Print and shaded views of the part. All mm, measured from the part's lowest x, y and z. Coordinates: 2 decimals unless noted, no trailing zeros. Order: outer loops, then holes, each group sorted by start corner. A loop starts at its lowest first (then second) coordinate and runs counter-clockwise, first axis right, second up. Notation, with made-up numbers: (-6, 85.25) -> (8, 85.25) arc R20 ccw to (8, 92.25) -> close; hole circle Ø2 at (87, -2.75). An arc over 180 degrees is marked (long way). Write item = value, one per line. Start each with the question number.
Q1. Cut at A-A, the plane z = 2.65. List the corners of the cut face in (x, y), plus the area to 3 significant figures.
Q2. Cut at C-C, the plane y = 20. List the corners of the cut face in (x, z).
Q3. Flat gauge pins, fed straight in: pin 1 (3 mm diameter, centred on x = 6.5, y = 7, fed in from +Z); pin 2 (1 mm diameter, centred on y = 12.5, z = 1.5, fed in from +X); pin 3 (3 mm diameter, centred on x = 38.5, y = 37, fed in from +Z); pin 4 (1 mm diameter, centred on x = 7, z = 3, fed in from +Y). Where does each tip first touch, or does it go through?
Q4. Cut at B-B, the plane x = 28. List the corners of the cut face in (y, z).
Q5. Wall check: line 1 (Z direction, x = 4.5, y = 4.5); line 2 (Y direction, x = 22, z = 2.8); line 3 (Y direction, x = 37, z = 2.15) (1 decimal). Give the ranges that are in metal, low to high. Write a range as from..to.
Q6. Cut at D-D, the plane y = 37.5. List the corners of the cut face in (x, z), plus the area to 3 significant figures.
Q7. Mould opens along Y. For the marked faces 1, 2 and 3 say: +Y half, -Y half, draft (parallel to the pull), parting line (faces both ways), or undercut.
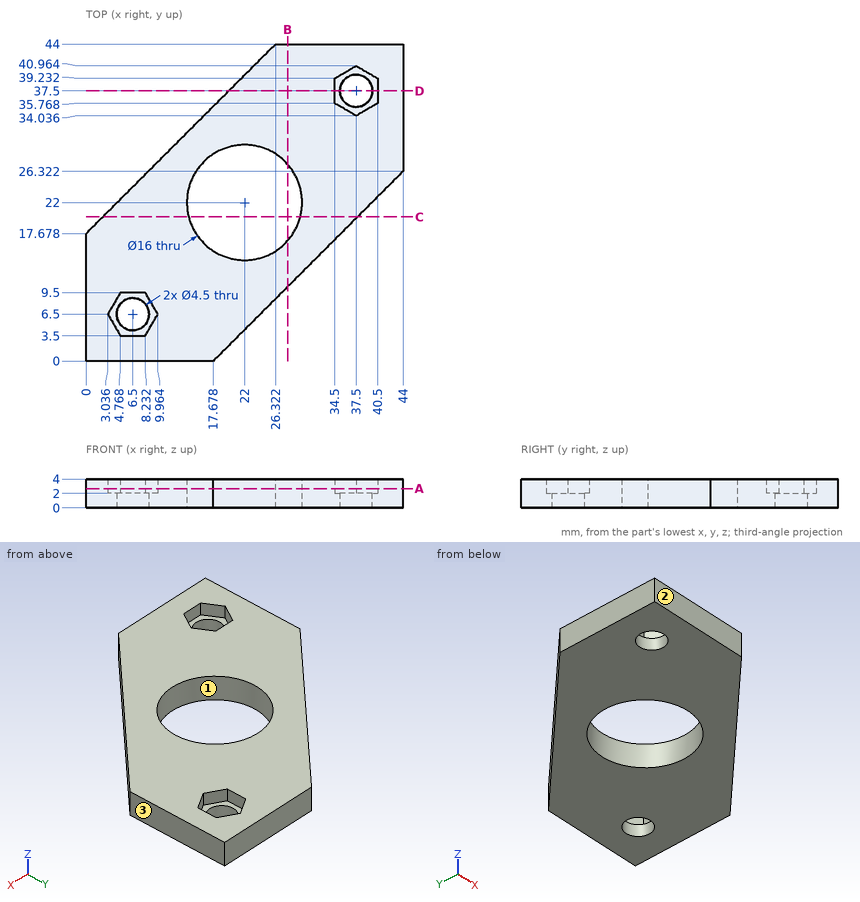
Here are the results:
q1.outline = (0, 0) -> (17.68, 0) -> (44, 26.32) -> (44, 44) -> (26.32, 44) -> (0, 17.68) -> close; hole (3.04, 6.5) -> (4.77, 3.5) -> (8.23, 3.5) -> (9.96, 6.5) -> (8.23, 9.5) -> (4.77, 9.5) -> close; hole circle Ø16 at (22, 22); hole (34.5, 35.77) -> (37.5, 34.04) -> (40.5, 35.77) -> (40.5, 39.23) -> (37.5, 40.96) -> (34.5, 39.23) -> close
q1.area = 980 mm²
q2.outline = (2.32, 0) -> (14.25, 0) -> (14.25, 4) -> (2.32, 4) -> close; (29.75, 0) -> (37.68, 0) -> (37.68, 4) -> (29.75, 4) -> close
q3.pin_1 = through
q3.pin_2 = 30.68
q3.pin_3 = 2
q3.pin_4 = 25.18
q4.outline = (10.32, 0) -> (16.71, 0) -> (16.71, 4) -> (10.32, 4) -> close; (27.29, 0) -> (44, 0) -> (44, 4) -> (27.29, 4) -> close
q5.line_1 = 0..2
q5.line_2 = 4.32..14, 30..39.68
q5.line_3 = 19.3..34.3, 40.7..44
q6.outline = (19.82, 0) -> (35.25, 0) -> (35.25, 2) -> (34.5, 2) -> (34.5, 4) -> (19.82, 4) -> close; (39.75, 0) -> (44, 0) -> (44, 4) -> (40.5, 4) -> (40.5, 2) -> (39.75, 2) -> close
q6.area = 75.7 mm²
q7.face_1 = undercut
q7.face_2 = -Y half
q7.face_3 = draft
